Geometry check sheet. Reference: drawing and pictorial views, mm from the part's lowest x, y, z. A direction names the side the tool comes from. Round coordinates to 2 decimals unless told otherwise and drop trailing zeros. Write each loop counter-clockwise with the first axis right and the second up, starting at its lowest first coordinate (ties: lowest second). Pieces come first, ordered by that corner, then holes. Notation, with made-up numbers: (44, 22.5) - (77, 22.5) arc R20 cw to (77, 26.5) - close; hole circle Ø8 at (18, 37). An arc over 180 degrees is marked (long way). Use one line per item in the form item = value. Start each with the question number.
1) Set-up check for the marked faces 1, 2 and 3: record each of +Z, -Z, +X, -X, +Y, -Y from which the full face is reachable in a straight line by a thin tool's end or side.
2) Scan lines: probe 1 along Y at (x, z) = (77, 7.75); probe 2 along X at (y, z) = (27, 2.75); probe 3 along X at (y, z) = (21.5, 8.75). Record each from-to range of solid material in increasing order.
3) Section check B-B (x = 64.5). Record the boundary of the cut face in (y, z), then the cut area to 3 significant figures.
4) Section check C-C (z = 12.75). Record the boundary of the cut face in (x, y), then the cut area to 3 significant figures.
5) Section check D-D (y = 42). Record the boundary of the cut face in (x, z).
6) Gauge pin test, flat ends, axial feed: P1, Ø16, axis at x = 41.5, y = 24, coming from the -Z side; P2, Ø5.5, axis at x = 77, y = 42, coming from the +Z side; P3, Ø1, axis at x = 70.5, z = 17, coming from the -Y side; P4, Ø5, axis at y = 24, z = 19, coming from the +X side. Record the tip position at first contact, or that the pin passes through.
7) Draft check along X on the marked faces 4, 5 and 6. Enter one of: +X half, -X half, draft (parallel to the pull), parting line (faces both ways), or undercut.
8) Section check A-A (y = 24). Record the boundary of the cut face in (x, z), then the cut area to 3 significant figures.
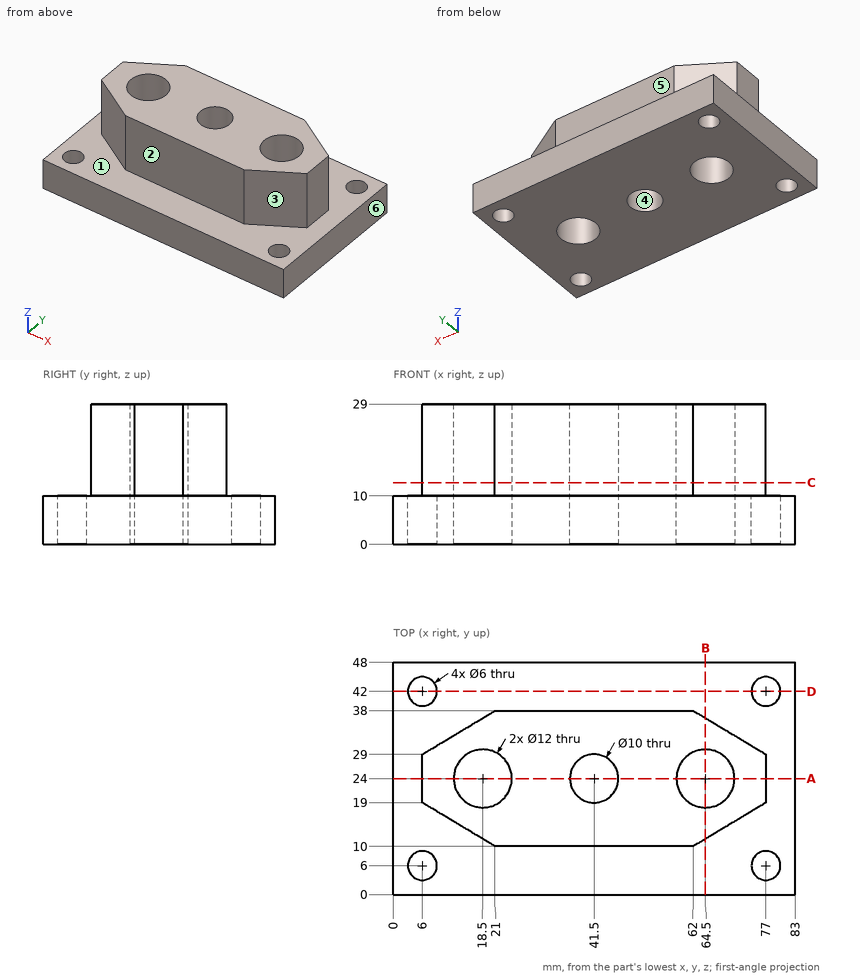
Results are:
q1.face_1 = +Z
q1.face_2 = +Z, +X, -X, -Y
q1.face_3 = +Z, +X, -Y
q2.probe_1 = 0 to 3, 9 to 39, 45 to 48
q2.probe_2 = 0 to 13.3, 23.7 to 37.5, 45.5 to 59.3, 69.7 to 83
q2.probe_3 = 0 to 13.05, 23.95 to 37.17, 45.83 to 59.05, 69.95 to 83
q3.outline = (0, 0) - (18, 0) - (18, 29) - (11.5, 29) - (11.5, 10) - (0, 10) - close; (30, 0) - (48, 0) - (48, 10) - (36.5, 10) - (36.5, 29) - (30, 29) - close
q3.area = 607 mm²
q4.outline = (6, 19) - (21, 10) - (62, 10) - (77, 19) - (77, 29) - (62, 38) - (21, 38) - (6, 29) - close; hole circle Ø12 at (18.5, 24); hole circle Ø10 at (41.5, 24); hole circle Ø12 at (64.5, 24)
q4.area = 1,410 mm²
q5.outline = (0, 0) - (3, 0) - (3, 10) - (0, 10) - close; (9, 0) - (74, 0) - (74, 10) - (9, 10) - close; (80, 0) - (83, 0) - (83, 10) - (80, 10) - close
q6.P1 = 0
q6.P2 = through
q6.P3 = 14.8
q6.P4 = 77
q7.face_4 = undercut
q7.face_5 = draft
q7.face_6 = +X half
q8.outline = (0, 0) - (12.5, 0) - (12.5, 29) - (6, 29) - (6, 10) - (0, 10) - close; (24.5, 0) - (36.5, 0) - (36.5, 29) - (24.5, 29) - close; (46.5, 0) - (58.5, 0) - (58.5, 29) - (46.5, 29) - close; (70.5, 0) - (83, 0) - (83, 10) - (77, 10) - (77, 29) - (70.5, 29) - close
q8.area = 1,190 mm²
